Autodesk Fusion 360 part; units mm, degrees
sketch "Sketch1" plane through (0, 0, 0) normal (0, 0, 1) x (1, 0, 0)
  line L0 (-30.479, 50.2485) -> (19.521, 50.2485)
  line L1 (19.521, 50.2485) -> (19.521, 0.2485)
  line L2 (19.521, 0.2485) -> (49.521, 0.2485)
  line L3 (-30.479, 50.2485) -> (-30.479, 80.2485)
  line L4 (-30.479, 80.2485) -> (49.521, 80.2485)
  line L5 (49.521, 80.2485) -> (49.521, 0.2485)
  line L6 (19.521, 0.2485) -> (22.521, 0.2485)
  line L7 (-30.479, 50.2485) -> (-30.479, 53.2485)
  line L8 (-30.479, 53.2485) -> (22.521, 53.2485)
  line L9 (22.521, 53.2485) -> (22.521, 0.2485)
  dimension "d1" = 50
  dimension "d2" = 50
  dimension "d3" = 30
  dimension "d4" = 30
  dimension "d5" = 80
  dimension "d6" = 3
  dimension "d7" = 3
  dimension "d8" = 53
extrude "Extrude1" add sketch "Sketch1" along normal blind 3 makes body 1
extrude "Extrude2" add sketch "Sketch1" along normal blind 60 separate body contours L0 L1 L2 L3 L6 L7 L8 L9 makes body 2
combine "Combine1" operation add target body 2 tool bodies 1
sketch "Sketch2" plane through (0, 0, 3) normal (0, 0, 1) x (-1, 0, 0)
  line L0 (30.479, -53.2485) -> (-22.521, -53.2485)
  line L1 (-22.521, -53.2485) -> (-22.521, -0.2485)
  line L2 (-22.521, -0.2485) -> (-49.521, -0.2485)
  line L3 (-49.521, -0.2485) -> (-49.521, -80.2485)
  line L4 (-49.521, -80.2485) -> (30.479, -80.2485)
  line L5 (30.479, -80.2485) -> (30.479, -53.2485)
  line L6 (-49.521, -0.2485) -> (-39.521, -0.2485)
  line L7 (-39.521, -0.2485) -> (-39.521, -25.2485)
  line L8 (30.479, -80.2485) -> (30.479, -70.2485)
  line L9 (30.479, -70.2485) -> (5.479, -70.2485)
  dimension "d13" = 10
  dimension "d14" = 25
  dimension "d15" = 10
  dimension "d16" = 25
hole "Hole1" at (39.521, 25.2485, 3) at (-5.479, 70.2485, 3) direction (0, 0, -1) diameter 4.2 end through all countersink diameter 8.6 countersink angle 90 bodies 2 2
sketch "Sketch3" plane through (22.521, 0, 0) normal (1, 0, 0) x (0, 1, 0)
  line L0 (0.2485, 3) -> (53.2485, 3)
  line L1 (53.2485, 3) -> (53.2485, 60)
  line L2 (53.2485, 60) -> (0.2485, 60)
  line L3 (0.2485, 60) -> (0.2485, 3)
  line L4 (0.2485, 3) -> (0.2485, 18)
  line L5 (0.2485, 18) -> (15.2485, 18)
  line L6 (53.2485, 60) -> (53.2485, 45)
  line L7 (53.2485, 45) -> (38.2485, 45)
  dimension "d22" = 15
  dimension "d23" = 15
  dimension "d24" = 15
  dimension "d25" = 15
hole "Hole2" at (22.521, 15.2485, 18) at (22.521, 38.2485, 45) direction (-1, 0, 0) diameter 4.2 end through all countersink diameter 8.6 countersink angle 90 bodies 2 2
sketch "Sketch4" plane through (0, 53.2485, 0) normal (0, 1, 0) x (-1, 0, 0)
  line L0 (-22.521, 3) -> (30.479, 3)
  line L1 (30.479, 3) -> (30.479, 60)
  line L2 (30.479, 60) -> (-22.521, 60)
  line L3 (-22.521, 60) -> (-22.521, 3)
  line L4 (-22.521, 3) -> (-22.521, 18)
  line L5 (-22.521, 18) -> (-7.521, 18)
  line L6 (30.479, 60) -> (30.479, 45)
  line L7 (30.479, 45) -> (15.479, 45)
  dimension "d31" = 15
  dimension "d32" = 15
  dimension "d33" = 15
  dimension "d34" = 15
hole "Hole3" at (-15.479, 53.2485, 45) at (7.521, 53.2485, 18) direction (0, -1, 0) diameter 4.2 end through all countersink diameter 8.6 countersink angle 90 bodies 2 2
fillet "Fillet1" radius 3 2 edges at (22.521, 53.2485, 31.5) (49.521, 80.2485, 1.5) on bodies 2
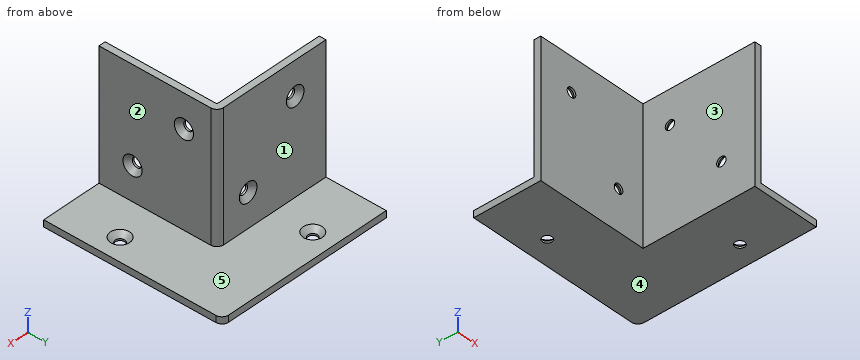
The listing builds one solid part. Answer for the finished solid, in the listing's coordinates (mm). Face numbers are marked on the shaded views. A direction names the side the tool comes from. Round coordinates to 2 decimals unless told otherwise and drop trailing zeros. Loops run counter-clockwise (first coordinate to the right, second up) from the corner with the lowest first, then second, coordinate; pieces in that order, holes last.
Q1. Which of the six approach directions +Z, -Z, +X, -X, +Y, -Y give full straight-line access (tool end or side, diameter ignored) to the marked faces 1, 2, 3, 4 and 5?
Q2. Given pin 1 Ø12 at (y, z) = (29, 34) entering from -X; pin 2 Ø25 at (x, z) = (-17, 27.5) entering from -Y; pin 3 Ø1.5 at (x, z) = (12, 7) entering from +Y, each flat-ended and moving along its own axis, determine where each tip first touches the part or whether it passes through.
Q3. Section A-A, the plane z = 45 is taken. Determine the outline of the cut face in (x, y).
Q4. Find the intervals of material crossed by line 1 (X direction, y = 50.4, z = 45); line 2 (Y direction, x = 19.7, z = 45); line 3 (X direction, y = 48.5, z = 26), in increasing order.
Q5. Section C-C, the plane z = 56 is taken. Determine the outline of the cut face in (x, y), then the cut area to 3 significant figures.
Q6. Section B-B, the plane y = 6.5 is taken. Determine the outline of the cut face in (x, z).
Completed:
1. face 1: +Z, +X, -X, +Y
1. face 2: +Z, +X, +Y, -Y
1. face 3: +Z, -Z, -X, -Y
1. face 4: -Z, +X, -X, +Y, -Y
1. face 5: +Z, +X, +Y
2. pin 1: stops at x = 19.52
2. pin 2: stops at y = 50.25
2. pin 3: stops at y = 53.25
3. outline: (-30.48, 50.25) - (-17.58, 50.25) - (-17.58, 51.05) - (-19.78, 53.25) - (-30.48, 53.25) - close; (-13.38, 50.25) - (19.52, 50.25) - (19.52, 40.35) - (20.32, 40.35) - (22.52, 42.55) - (22.52, 50.25) arc R3 ccw to (19.52, 53.25) - (-11.18, 53.25) - (-13.38, 51.05) - close; (19.52, 0.25) - (22.52, 0.25) - (22.52, 33.95) - (20.32, 36.15) - (19.52, 36.15) - close
4. line 1: x = -30.48 to -17.58, -13.38 to 22.52
4. line 2: y = 0.25 to 36.15, 40.35 to 53.24
4. line 3: x = 19.52 to 22.52
5. outline: (-30.48, 50.25) - (19.52, 50.25) - (19.52, 0.25) - (22.52, 0.25) - (22.52, 50.25) arc R3 ccw to (19.52, 53.25) - (-30.48, 53.25) - close
5. area: 307 mm2
6. outline: (19.52, 0) - (49.52, 0) - (49.52, 3) - (22.52, 3) - (22.52, 60) - (19.52, 60) - close
